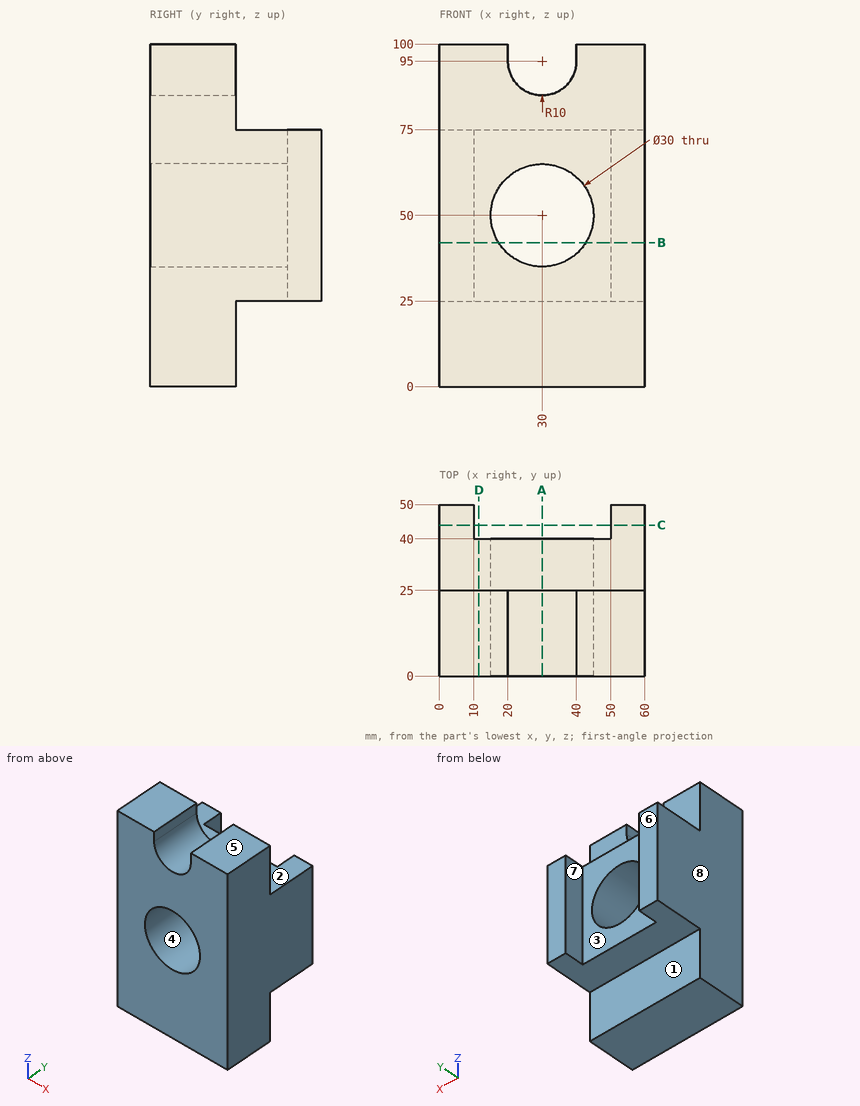
Answer from the drawing. Dimensions are ordinates in mm from the lowest x, y and z of the part. A direction names the side the tool comes from. Give positions to 0.01 mm unless a question says otherwise; leave off trailing zeros. Order: outer loops, then holes, each group sorted by start corner. A loop starts at its lowest first (then second) coordinate and runs counter-clockwise, first axis right, second up. Notation, with made-up numbers: (5.5, -3) - (55.5, -3) arc R27 ccw to (55.5, 23) - close; hole circle Ø4 at (29.5, -21.5). An arc over 180 degrees is marked (long way). One line per item, written item: value. Start each with the question number.
1) Find the intervals of material crossed by L1, parallel to X at y = 26, z = 50; L2, parallel to X at y = 43, z = 29; L3, parallel to Y at x = 46.5, z = 29, in increasing order.
2) A cutting plane is placed at B-B on z = 42. Give the vertices of the cut face in (x, y).
3) The mould has two halves that part along X. Classify the marked faces 6, 7 and 8: released by +X, released by -X, zero draft, split by the parting line, or undercut.
4) A cutting plane is placed at D-D on x = 11.5. Give the vertices of the cut face in (y, z), then the cut area to 3 significant figures.
5) A cutting plane is placed at C-C on y = 44. Give the vertices of the cut face in (x, z), then the cut area to 3 significant figures.
6) A cutting plane is placed at A-A on x = 30. Give the vertices of the cut face in (y, z).
7) A tool of negligible diameter and unlimited length cuts with its end or side. For the marked faces 1, 2, 3, 4 and 5, from which of +Z, -Z, +X, -X, +Y, -Y can it reach the whole face along a straight path? Write none if from no direction.
8) Given pin 1 Ø12.5 at (x, y) = (22.5, 40) entering from +Z; pin 2 Ø6 at (y, z) = (20.5, 27) entering from -X; pin 3 Ø1 at (x, y) = (36.5, 37.5) entering from -Z; pin 4 Ø20 at (x, z) = (20, 92) entering from +Y, each flat-ended and moving along its own axis, determine where each tip first touches the part or whether it passes through.
Answer sheet:
1. L1: x = 0 to 15, 45 to 60
1. L2: x = 0 to 10, 50 to 60
1. L3: y = 0 to 40
2. outline: (0, 0) - (17.31, 0) - (17.31, 40) - (10, 40) - (10, 50) - (0, 50) - close; (42.69, 0) - (60, 0) - (60, 50) - (50, 50) - (50, 40) - (42.69, 40) - close
3. face 6: zero draft
3. face 7: undercut
3. face 8: released by -X
4. outline: (0, 0) - (25, 0) - (25, 25) - (40, 25) - (40, 75) - (25, 75) - (25, 100) - (0, 100) - close
4. area: 3,250 mm2
5. outline: (0, 25) - (10, 25) - (10, 75) - (0, 75) - close; (50, 25) - (60, 25) - (60, 75) - (50, 75) - close
5. area: 1,000 mm2
6. outline: (0, 0) - (25, 0) - (25, 25) - (40, 25) - (40, 35) - (0, 35) - close; (0, 65) - (40, 65) - (40, 75) - (25, 75) - (25, 85) - (0, 85) - close
7. face 1: -Z, +X, -X, +Y
7. face 2: +Z, +X, -X, +Y
7. face 3: +Z, -Z, +Y
7. face 4: +Y, -Y
7. face 5: +Z, +X, -X, +Y, -Y
8. pin 1: stops at z = 75
8. pin 2: stops at x = 0
8. pin 3: stops at z = 25
8. pin 4: stops at y = 25
